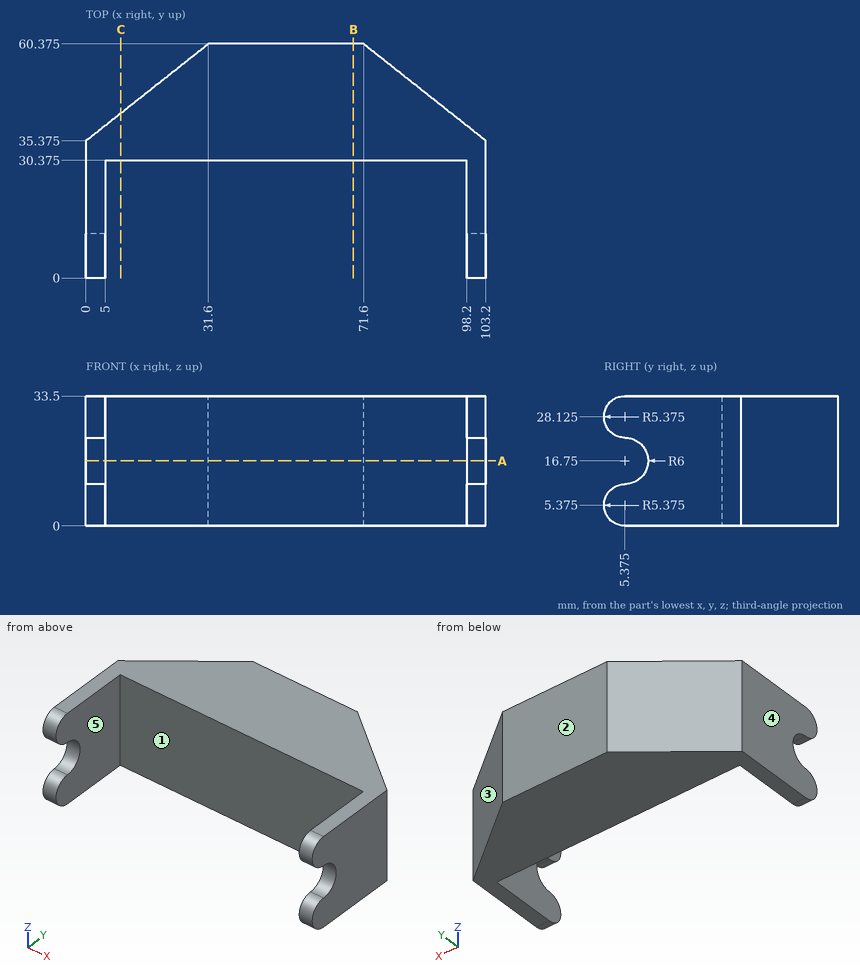
Input: dimensioned drawing with shaded views. Units: mm. Origin: part minimum x, y, z. A direction names the side the tool comes from. Round coordinates to 2 decimals unless told otherwise and drop trailing zeros. Order: outer loops, then holes, each group sorted by start corner. A loop starts at its lowest first (then second) coordinate and runs counter-clockwise, first axis right, second up.
1. Cut plane B-B, the plane x = 69. Output: boundary loops of the cut face in (y, z) (3 decimals).
The answers:
outline: (30.375, 0) - (60.375, 0) - (60.375, 33.5) - (30.375, 33.5) - close
2. Mould query, pull axis X, two halves, no side actions, for the marked faces 3, 4 and 5. Classes: released by +X, released by -X, zero draft, split by the parting line, or undercut.
The answers:
face 3: released by +X
face 4: released by -X
face 5: undercut
3. Material intervals for line 1 (X direction, y = 28, z = 30.5); line 2 (Y direction, x = 62, z = 4) (3 decimals); line 3 (Y direction, x = 19, z = 9) (3 decimals), sorted ascending.
The answers:
line 1: x = 0 to 5, 98.2 to 103.2
line 2: y = 30.375 to 60.375
line 3: y = 30.375 to 50.407
4. Cut plane C-C, the plane x = 9. Output: boundary loops of the cut face in (y, z) (3 decimals), then the cut area to 3 significant figures.
The answers:
outline: (30.375, 0) - (42.495, 0) - (42.495, 33.5) - (30.375, 33.5) - close
area: 406 mm2
5. Cut plane A-A, the plane z = 16.75. Output: boundary loops of the cut face in (x, y) (3 decimals).
The answers:
outline: (0, 11.375) - (5, 11.375) - (5, 30.375) - (98.2, 30.375) - (98.2, 11.375) - (103.2, 11.375) - (103.2, 35.375) - (71.6, 60.375) - (31.6, 60.375) - (0, 35.375) - close
6. Pin query (flat end, axial travel): P1, Ø10, axis at y = 47.5, z = 23, coming from the +X side; P2, Ø10, axis at y = 54, z = 23.5, coming from the -X side; P3, Ø10, axis at x = 55.5, z = 12, coming from the -Y side (3 decimals). Return the tip coordinate at first contact, or that it passes through.
The answers:
P1: stops at x = 94.19
P2: stops at x = 17.22
P3: stops at y = 30.375
7. Set-up query: the marked faces 1 and 2. Return all of +Z, -Z, +X, -X, +Y, -Y with unobstructed straight access to the full face (end or side cutting, diameter ignored); none if empty.
The answers:
face 1: +Z, -Z, -Y
face 2: +Z, -Z, +X, -X, +Y
